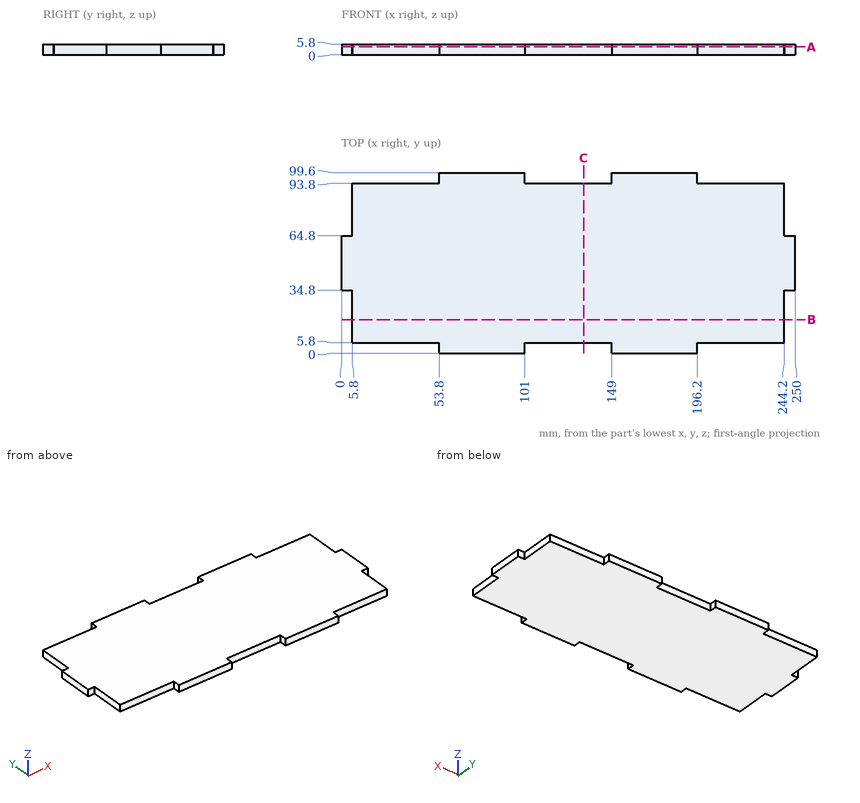
Job drawing, mm, ordinate dimensions from the low corner. One solid piece. Coordinates: 2 decimals unless noted, no trailing zeros. Write each loop counter-clockwise with the first axis right and the second up, starting at its lowest first coordinate (ties: lowest second). Pieces come first, ordered by that corner, then holes. Notation, with made-up numbers: M -7,72.5 L 51,72.5 A20 cw 51,76.5 Z; hole C -23,-38 d8. An arc over 180 degrees is marked long. Answer as a JSON object with one key per item and string values. Group by question number.
1) Pin check, flat tips, straight feed: pin 1 Ø1.7 at (y, z) = (3, 2) entering from -X; pin 2 Ø1.7 at (x, z) = (2, 2.5) entering from +Y; pin 3 Ø2 at (y, z) = (86, 2.5) entering from -X. Stop position of each tip, or through.
2) Saw through at B-B (y = 18.5). Write the cut outline in (x, z), plus the area to 3 significant figures.
3) Saw through at C-C (x = 133.5). Write the cut outline in (y, z), plus the area to 3 significant figures.
4) Saw through at A-A (z = 4.15). Write the cut outline in (x, y), plus the area to 3 significant figures.
5) Wall check: line 1 (Y direction, x = 47.5, z = 4.55); line 2 (X direction, y = 31.5, z = 0.3); line 3 (X direction, y = 94, z = 4.7). Give the ranges that are in metal, low to high. Write a range as from..to.
Values follow:
{
 "1": {"pin 1": "stops at x = 53.8", "pin 2": "stops at y = 64.8", "pin 3": "stops at x = 5.8"},
 "2": {"outline": "M 5.8,0 L 244.2,0 L 244.2,5.8 L 5.8,5.8 Z", "area": "1,380 mm2"},
 "3": {"outline": "M 5.8,0 L 93.8,0 L 93.8,5.8 L 5.8,5.8 Z", "area": "510 mm2"},
 "4": {"outline": "M 0,34.8 L 5.8,34.8 L 5.8,5.8 L 53.8,5.8 L 53.8,0 L 101,0 L 101,5.8 L 149,5.8 L 149,0 L 196.2,0 L 196.2,5.8 L 244.2,5.8 L 244.2,34.8 L 250,34.8 L 250,64.8 L 244.2,64.8 L 244.2,93.8 L 196.2,93.8 L 196.2,99.6 L 149,99.6 L 149,93.8 L 101,93.8 L 101,99.6 L 53.8,99.6 L 53.8,93.8 L 5.8,93.8 L 5.8,64.8 L 0,64.8 Z", "area": "22,400 mm2"},
 "5": {"line 1": "y = 5.8..93.8", "line 2": "x = 5.8..244.2", "line 3": "x = 53.8..101, 149..196.2"}
}
